Verification items for the finished model (mm, model axes). A direction names the side the tool comes from. Round coordinates to 2 decimals unless told otherwise and drop trailing zeros. Loops run counter-clockwise (first coordinate to the right, second up) from the corner with the lowest first, then second, coordinate; pieces in that order, holes last. Notation, with made-up numbers: (3.5, -4.75) -> (47.5, -4.75) arc R29 ccw to (47.5, 24.25) -> close; hole circle Ø6 at (3, 21). An arc over 180 degrees is marked (long way). Write item = value, one per line.
```python
from build123d import *

# Parameters (mm, degrees)
SKETCH1_W           = 130
SKETCH1_H           = 20
BOSS_EXTRUDE1_DEPTH = 4.9
SKETCH3_W           = 4.9
SKETCH3_H           = 4.9
BOSS_EXTRUDE2_DEPTH = 20
SKETCH4_W           = 130
SKETCH4_H           = 4
BOSS_EXTRUDE3_DEPTH = 7.5
SKETCH5_W           = 7.3
SKETCH5_H           = 3.8
BOSS_EXTRUDE4_DEPTH = 4.9
SKETCH6_W           = 7.3
SKETCH6_H           = 3.8
BOSS_EXTRUDE5_DEPTH = 4.9


with BuildPart() as part:
    # Sketch1 → Boss-Extrude1 (new body)
    with BuildSketch(Plane.XY):
        with Locations((7.416107383, 21.263982103)):
            Rectangle(SKETCH1_W, SKETCH1_H)
    extrude(amount=BOSS_EXTRUDE1_DEPTH)

    # Sketch3 → Boss-Extrude2 (add)
    with BuildSketch(Plane(origin=(72.416107383, 0, 0), x_dir=(0, 0, -1), z_dir=(1, 0, 0))):
        with Locations((-2.45, 28.813982103)):
            Rectangle(SKETCH3_W, SKETCH3_H)
    boss_extrude2 = extrude(amount=BOSS_EXTRUDE2_DEPTH)

    # Mirror1: Boss-Extrude2 across plane
    add(boss_extrude2.mirror(Plane.ZY.offset(-7.416107383)))

    # Sketch4 → Boss-Extrude3 (add)
    with BuildSketch(Plane(origin=(0, 0, 0), x_dir=(-1, 0, 0), z_dir=(0, 0, -1))):
        with Locations((-7.416107383, 13.263982103)):
            Rectangle(SKETCH4_W, SKETCH4_H)
    extrude(amount=BOSS_EXTRUDE3_DEPTH)

    # Sketch5 → Boss-Extrude4 (add)
    with BuildSketch(Plane.XZ.offset(-11.263982103)):
        with Locations((28.666107383, 3)):
            Rectangle(SKETCH5_W, SKETCH5_H)
    boss_extrude4 = extrude(amount=BOSS_EXTRUDE4_DEPTH)

    # Mirror2: Boss-Extrude4 across plane
    add(boss_extrude4.mirror(Plane.ZY.offset(-7.416107383)))

    # Sketch6 → Boss-Extrude5 (add)
    with BuildSketch(Plane.XZ.offset(-11.263982103)):
        with Locations((58.666107383, 3)):
            Rectangle(SKETCH6_W, SKETCH6_H)
    boss_extrude5 = extrude(amount=BOSS_EXTRUDE5_DEPTH)

    # Mirror3: Boss-Extrude5 across plane
    add(boss_extrude5.mirror(Plane.ZY.offset(-7.416107383)))


solid = part.part
```
(1) Draft check along X on faces 1 (the face through (9, 31.264, 2)), 2 (the face through (55.016, 9, 3)), 3 (the face through (-17.484, 9, 3)), 4 (the face through (-47.484, 9, 3)). Enter one of: released by +X, released by -X, zero draft, split by the parting line, or undercut.
Filled sheet:
face_1 = zero draft
face_2 = undercut
face_3 = undercut
face_4 = released by -X
(2) Sectioned sample at D-D, the plane x = 80.5. Record the cut outline in (y, z), and give its area (3 significant figures).
Filled sheet:
outline = (26.36, 0) -> (31.26, 0) -> (31.26, 4.9) -> (26.36, 4.9) -> close
area = 24.0 mm2
(3) Material ranges on probe 1 along Z at (x, y) = (59, 7.75); probe 2 along Z at (x, y) = (4.5, 26); probe 3 along Y at (x, z) = (-30, -3), recorded low to high. Write a range as from..to.
Filled sheet:
probe_1 = 1.1..4.9
probe_2 = 0..4.9
probe_3 = 11.26..15.26
(4) Sectioned sample at B-B, the plane x = -12. Record the cut outline in (y, z).
Filled sheet:
outline = (6.36, 1.1) -> (11.26, 1.1) -> (11.26, -7.5) -> (15.26, -7.5) -> (15.26, 0) -> (31.26, 0) -> (31.26, 4.9) -> (6.36, 4.9) -> close
(5) Sectioned sample at A-A, the plane z = 2.5. Record the cut outline in (x, y).
Filled sheet:
outline = (-77.58, 26.36) -> (-57.58, 26.36) -> (-57.58, 11.26) -> (-47.48, 11.26) -> (-47.48, 6.36) -> (-40.18, 6.36) -> (-40.18, 11.26) -> (-17.48, 11.26) -> (-17.48, 6.36) -> (-10.18, 6.36) -> (-10.18, 11.26) -> (25.02, 11.26) -> (25.02, 6.36) -> (32.32, 6.36) -> (32.32, 11.26) -> (55.02, 11.26) -> (55.02, 6.36) -> (62.32, 6.36) -> (62.32, 11.26) -> (72.42, 11.26) -> (72.42, 26.36) -> (92.42, 26.36) -> (92.42, 31.26) -> (-77.58, 31.26) -> close
(6) Go/stop test with flat-tipped pins: pin 1 Ø13 at (x, y) = (42, 27) entering from -Z; pin 2 Ø3 at (y, z) = (9, 3) entering from -X; pin 3 Ø1.5 at (y, z) = (19.5, 2) entering from -X. Record where each tip stops, or that it passes through.
Filled sheet:
pin_1 = 0
pin_2 = -47.48
pin_3 = -57.58
(7) Set-up check for faces 5 (the face through (29, 6.364, 3)), 6 (the face through (92.416, 29, 2)), 7 (the face through (9, 23, 0)), 8 (the face through (62.316, 9, 3)), 9 (the face through (59, 9, 1.1)): record each of +Z, -Z, +X, -X, +Y, -Y from which the full face is reachable in a straight line by a thin tool's end or side.
Filled sheet:
face_5 = +Z, -Z, +X, -X, -Y
face_6 = +Z, -Z, +X, +Y, -Y
face_7 = -Z, +X, -X, +Y
face_8 = +Z, -Z, +X, -Y
face_9 = -Z, +X, -X, -Y
(8) Sectioned sample at C-C, the plane y = 13.25. Record the cut outline in (x, z), and give its area (3 significant figures).
Filled sheet:
outline = (-57.58, -7.5) -> (72.42, -7.5) -> (72.42, 4.9) -> (-57.58, 4.9) -> close
area = 1,610 mm2
